from build123d import *

# Parameters (mm, degrees)
SKETCH1_W           = 37.5
SKETCH1_H           = 16.7
BOSS_EXTRUDE1_DEPTH = 3.2
SKETCH2_W           = 8.6
SKETCH2_H           = 8.6
SKETCH2_W_2         = 6.8
SKETCH2_W_3         = 3.2
SKETCH2_H_2         = 2.5
BOSS_EXTRUDE2_DEPTH = 1.1
BOSS_EXTRUDE3_DEPTH = 0.1
SKETCH4_W           = 2.5
SKETCH4_H           = 10.3
BOSS_EXTRUDE4_DEPTH = 2.5
SKETCH5_W           = 2.5
SKETCH5_H           = 0.1
CUT_EXTRUDE1_DEPTH  = 0.2
SKETCH6_W           = 0.7
SKETCH6_H           = 0.7


with BuildPart() as part:
    # Sketch1 → Boss-Extrude1 (new body)
    with BuildSketch(Plane(origin=(0, 0, 0), x_dir=(1, 0, 0), z_dir=(0, 1, 0))):
        Rectangle(SKETCH1_W, SKETCH1_H)
    extrude(amount=BOSS_EXTRUDE1_DEPTH)

    # Sketch2 → Boss-Extrude2 (add)
    with BuildSketch(Plane(origin=(0, 3.2, 0), x_dir=(1, 0, 0), z_dir=(0, 1, 0))):
        with Locations((-4.05, 1.85)):
            Rectangle(SKETCH2_W, SKETCH2_H)
        with Locations((5.15, 1.85)):
            Rectangle(SKETCH2_W_2, SKETCH2_H)
        with Locations((-7.25, -4.2)):
            Rectangle(SKETCH2_W_3, SKETCH2_H_2)
    extrude(amount=BOSS_EXTRUDE2_DEPTH)

    # Sketch3 → Boss-Extrude3 (add)
    with BuildSketch(Plane(origin=(0, 3.2, 0), x_dir=(1, 0, 0), z_dir=(0, 1, 0))):
        Polygon((-14.05, 6.55), (-18.25, 6.55), (-18.25, 4.35), (-15.75, 4.35), (-15.75, 3.6), (-18.25, 3.6), (-18.25, 1.4), (-15.75, 1.4), (-15.75, 0.65), (-18.25, 0.65), (-18.25, -1.55), (-15.75, -1.55), (-15.75, -2.3), (-18.25, -2.3), (-18.25, -4.5), (-15.75, -4.5), (-15.75, -5.25), (-18.25, -5.25), (-18.25, -6.55), (-17.5, -6.55), (-17.5, -6), (-15, -6), (-15, -3.8), (-17.5, -3.8), (-17.5, -3.05), (-15, -3.05), (-15, -0.85), (-17.5, -0.85), (-17.5, -0.1), (-15, -0.1), (-15, 2.1), (-17.5, 2.1), (-17.5, 2.85), (-15, 2.85), (-15, 5.05), (-17.5, 5.05), (-17.5, 5.8), (-14.05, 5.8), align=None)
    extrude(amount=BOSS_EXTRUDE3_DEPTH)

    # Sketch4 → Boss-Extrude4 (add)
    with BuildSketch(Plane(origin=(0, 3.2, 0), x_dir=(1, 0, 0), z_dir=(0, 1, 0))):
        with Locations((17.4, 0)):
            Rectangle(SKETCH4_W, SKETCH4_H)
    extrude(amount=BOSS_EXTRUDE4_DEPTH)

    # Sketch5 → Cut-Extrude1 (cut)
    with BuildSketch(Plane(origin=(0, 5.7, 0), x_dir=(1, 0, 0), z_dir=(0, 1, 0))):
        with Locations((17.4, 2.6)):
            Rectangle(SKETCH5_W, SKETCH5_H)
        with Locations((17.4, -2.6)):
            Rectangle(SKETCH5_W, SKETCH5_H)
        with Locations((17.4, 0)):
            Rectangle(SKETCH5_W, SKETCH5_H)
    extrude(amount=-CUT_EXTRUDE1_DEPTH, mode=Mode.SUBTRACT)

    # Sweep1: sweep along a path in Sketch7
    with BuildLine(Plane.XY) as sweep1_path:
        Line((17.4, 5.7), (17.4, 6.75))
        ThreePointArc((17.4, 6.75), (17.605025253, 7.244974747), (18.1, 7.45))
        Line((18.1, 7.45), (25.15, 7.45))
    # Sketch6 → Sweep1 (sweep)
    with BuildSketch(Plane(origin=(0, 5.7, 0), x_dir=(1, 0, 0), z_dir=(0, 1, 0))):
        with Locations((17.4, 3.9)):
            Rectangle(SKETCH6_W, SKETCH6_H)
        with Locations((17.4, 1.3)):
            Rectangle(SKETCH6_W, SKETCH6_H)
        with Locations((17.4, -1.3)):
            Rectangle(SKETCH6_W, SKETCH6_H)
        with Locations((17.4, -3.9)):
            Rectangle(SKETCH6_W, SKETCH6_H)
    sweep(path=sweep1_path.line)


solid = part.part
Source: CAD feature listing. Evaluate the final solid. Frame: model axes, mm. A direction names the side the tool comes from. Coordinates: 2 decimals unless noted, no trailing zeros. Order: outer loops, then holes, each group sorted by start corner. A loop starts at its lowest first (then second) coordinate and runs counter-clockwise, first axis right, second up. Notation, with made-up numbers: M 45,-35 L 82,-35 A29 cw 82,-14 Z; hole C 88,11.5 d10. An arc over 180 degrees is marked long. Write each question's results on one line, items separated by ' | '. Start each with the question number.
Item 1: Draft query along Y for faces 1 (the face through (-16.6, 3.3, -0.1)), 2 (the face through (18, 5.7, 1)), 3 (the face through (-7, 4, 2.95)). Return one class per face: pulls with the +Y half, pulls with the -Y half, needs draft (parallel to the pull), parting line crosses it, or undercut.
Item 2: Cut plane C-C (z = -7). Return loops of the section in (x, y), and give its area (3 significant figures).
Item 3: Cut plane D-D (y = 1.25). Return loops of the section in (x, z), and give its area (3 significant figures).
Item 4: Cut plane A-A (y = 6.25). Return loops of the section in (x, z), and give its area (3 significant figures).
Item 5: First-contact query: pin 1 Ø0.6 at (y, z) = (4, 3.5) entering from +X; pin 2 Ø10 at (x, z) = (1, 1.5) entering from -Y; pin 3 Ø5 at (x, z) = (7, 4.5) entering from +Y; pin 4 Ø0.6 at (x, y) = (20.5, 6.5) entering from +Z. Flat tips, straight axial feed; report the tip coordinate or a pass-through.
Item 6: Set-up query: faces 4 (the face through (17, 4, -5.15)), 5 (the face through (20.1, 7.5, -0.95)), 6 (the face through (8.55, 4, -2)). Return all of +Z, -Z, +X, -X, +Y, -Y with unobstructed straight access to the full face (end or side cutting, diameter ignored); none if empty.
Item 7: Line query: probe 1 along X at (y, z) = (4, -0.5); probe 2 along X at (y, z) = (0.5, 1.5); probe 3 along Y at (x, z) = (-13, 6). Output: solid intervals per line, ascending.
Item 8: Cut plane B-B (x = 6.5). Return loops of the section in (y, z), and give its area (3 significant figures).
Checked values:
1) face 1: pulls with the +Y half | face 2: undercut | face 3: needs draft
2) outline: M -18.75,0 L 18.75,0 L 18.75,3.2 L -18.75,3.2 Z | area: 120 mm2
3) outline: M -18.75,-8.35 L 18.75,-8.35 L 18.75,8.35 L -18.75,8.35 Z | area: 626 mm2
4) outline: M 17.05,-4.25 L 17.75,-4.25 L 17.75,-3.55 L 17.05,-3.55 Z; M 17.05,-1.65 L 17.75,-1.65 L 17.75,-0.95 L 17.05,-0.95 Z; M 17.05,0.95 L 17.75,0.95 L 17.75,1.65 L 17.05,1.65 Z; M 17.05,3.55 L 17.75,3.55 L 17.75,4.25 L 17.05,4.25 Z | area: 1.96 mm2
5) pin 1: stops at x = 18.65 | pin 2: stops at y = 0 | pin 3: stops at y = 4.3 | pin 4: passes through
6) face 4: -Z, +X, +Y | face 5: +X, -X, +Y | face 6: +Z, -Z, +Y
7) probe 1: x = -8.35 to 0.25, 1.75 to 8.55, 16.15 to 18.65 | probe 2: x = -18.75 to 18.75 | probe 3: y = 0 to 3.2
8) outline: M 0,-8.35 L 3.2,-8.35 L 3.2,-6.15 L 4.3,-6.15 L 4.3,2.45 L 3.2,2.45 L 3.2,8.35 L 0,8.35 Z | area: 62.9 mm2
